Read the model definition and answer for the solid it produces. Units are mm, in the model's axes. A direction names the side the tool comes from. Give positions to 0.01 mm unless a question says otherwise; leave off trailing zeros. Loops run counter-clockwise (first coordinate to the right, second up) from the corner with the lowest first, then second, coordinate; pieces in that order, holes last. Notation, with made-up numbers: (69, 6) -> (126, 6) arc R16 cw to (126, 13) -> close; hole circle Ø8 at (89.5, -3.75). An arc over 180 degrees is marked (long way). Return JSON: item names as keys, results as strings. Group by question number.
from build123d import *

# Parameters (mm, degrees)
F0_R     = 4.25
F1_DEPTH = 3
F2_R     = 5
F3_R     = 6
F4_R     = 1
F5_SIZE  = 1


with BuildPart() as f1:
    # F0 (on Top) → F1 (new body)
    with BuildSketch(Plane.XY):
        with BuildLine():
            Line((-62.1857971695, 22.9072221785), (-52.3882933556, 32.7997051499))
            ThreePointArc((-52.3882933556, 32.7997051499), (-50.9844964361, 40.1186300293), (-48.1611355423, 47.0154365688))
            Line((-48.1611355423, 47.0154365688), (-69.9716899396, 24.9934458586))
            Line((-69.9716899396, 24.9934458586), (-62.1857971695, 22.9072221785))
        make_face()
        with BuildLine():
            ThreePointArc((-48.1611355423, 47.0154365688), (-50.9844964361, 40.1186300293), (-52.3882933556, 32.7997051499))
            Line((-52.3882933556, 32.7997051499), (-34.5789852905, 50.7816605657))
            ThreePointArc((-34.5789852905, 50.7816605657), (-28.0931597891, 55.634884838), (-20.47471121, 58.3878758514))
            ThreePointArc((-20.47471121, 58.3878758514), (-20.102300057, 64.1509445203), (-15.0399766137, 66.9302487327))
            ThreePointArc((-15.0399766137, 66.9302487327), (-34.3636079514, 61.5681900471), (-48.1611355423, 47.0154365688))
        make_face()
        with BuildLine():
            ThreePointArc((-15.0399766137, 66.9302487327), (-20.102300057, 64.1509445203), (-20.47471121, 58.3878758514))
            ThreePointArc((-20.47471121, 58.3878758514), (-17.7708422565, 58.794319571), (-15.0399766285, 58.9302487327))
            ThreePointArc((-15.0399766285, 58.9302487327), (-12.3091109856, 58.7943195724), (-9.6052420174, 58.3878758514))
            ThreePointArc((-9.6052420174, 58.3878758514), (-9.1829975469, 59.628021329), (-9.0399766137, 60.9302487327))
            ThreePointArc((-9.0399766137, 60.9302487327), (-10.7973359266, 65.1728894198), (-15.0399766137, 66.9302487327))
        make_face()
        with BuildLine():
            ThreePointArc((-13.0399766137, 60.9302487327), (-13.6257630566, 59.5160351651), (-15.0399766285, 58.9302487327))
            ThreePointArc((-15.0399766285, 58.9302487327), (-16.4541901709, 62.3444623003), (-13.0399766137, 60.9302487327))
        make_face(mode=Mode.SUBTRACT)
        with BuildLine():
            ThreePointArc((-15.0399766285, 58.9302487327), (-17.7708422565, 58.794319571), (-20.47471121, 58.3878758514))
            ThreePointArc((-20.47471121, 58.3878758514), (-15.0399766137, 54.9302487327), (-9.6052420174, 58.3878758514))
            ThreePointArc((-9.6052420174, 58.3878758514), (-12.3091109856, 58.7943195724), (-15.0399766285, 58.9302487327))
        make_face()
        with BuildLine():
            ThreePointArc((1.4030809655, 2.8767422936), (1.5045728658, 0.9401614715), (3.2006690581, 0))
            Line((3.2006690581, 0), (8.2003000527, 0))
            ThreePointArc((8.2003000527, 0), (17.7947523333, 11.3158739167), (22.25, 25.4669616943))
            ThreePointArc((22.25, 25.4669616943), (22.40748073, 27.4458247627), (22.4600233863, 29.4302487327))
            ThreePointArc((22.4600233863, 29.4302487327), (11.4765276808, 55.9467530272), (-15.0399766137, 66.9302487327))
            ThreePointArc((-15.0399766137, 66.9302487327), (-10.7973359266, 65.1728894198), (-9.0399766137, 60.9302487327))
            ThreePointArc((-9.0399766137, 60.9302487327), (-9.1829975469, 59.628021329), (-9.6052420174, 58.3878758514))
            ThreePointArc((-9.6052420174, 58.3878758514), (6.2403570467, 48.8485551745), (12.4600233863, 31.4302487327))
            ThreePointArc((12.4600233863, 31.4302487327), (12.0822423248, 26.8876459708), (10.9592786697, 22.4698511575))
            ThreePointArc((10.9592786697, 22.4698511575), (9.6768596595, 19.375042196), (8.0276528973, 16.4591275743))
            Line((8.0276528973, 16.4591275743), (1.4030809655, 2.8767422936))
        make_face()
        with BuildLine():
            ThreePointArc((22.25, 25.4669616943), (17.7947523333, 11.3158739167), (8.2003000527, 0))
            Line((8.2003000527, 0), (29.5, 0))
            ThreePointArc((29.5, 0), (37.5, 8), (29.5, 16))
            Line((29.5, 16), (27.25, 16))
            ThreePointArc((27.25, 16), (23.7144660941, 17.4644660941), (22.25, 21))
            Line((22.25, 21), (22.25, 22.4049843981))
            Line((22.25, 22.4049843981), (22.25, 25.4669616943))
        make_face()
        with Locations((29.5, 8)):
            Circle(F0_R, mode=Mode.SUBTRACT)
    extrude(amount=F1_DEPTH)

    # F2
    f2_edges = [f1.edges().sort_by_distance(p)[0] for p in [
        (-20.474711, 58.387876, 1.5),
        (-9.605242, 58.387876, 1.5),
    ]]
    fillet(f2_edges, radius=F2_R)

    # F3
    f3_edges = [f1.edges().sort_by_distance(p)[0] for p in [
        (22.25, 25.466962, 1.5),
    ]]
    fillet(f3_edges, radius=F3_R)

    # F4
    f4_edges = [f1.edges().sort_by_distance(p)[0] for p in [
        (-69.97169, 24.993446, 1.5),
        (-62.185797, 22.907222, 1.5),
    ]]
    fillet(f4_edges, radius=F4_R)

    # F5
    f5_edges = [f1.edges().sort_by_distance(p)[0] for p in [
        (25.25, 8, 3),
        (25.25, 8, 0),
    ]]
    chamfer(f5_edges, length=F5_SIZE)


solid = f1.part
1. Straight lines are drawn through the part: line 1 (Y direction, x = 29.5, z = 1.25); line 2 (X direction, y = 60, z = 2.3); line 3 (X direction, y = 32, z = 2.5). For each, find the intervals that lie inside material, in ascending order. Write a range as from..to.
2. Section A-A on x = 6 is taken. Determine the outline of the cut face in (y, z), then the cut area to 3 significant figures.
3. Which of the six approach directions +Z, -Z, +X, -X, +Y, -Y give full straight-line access (tool end or side, diameter ignored) to faces 1 (the cylindrical face through (26.13, 5.41, 1.49)), 2 (the flat face through (16, 0, 1)), 3 (the cylindrical face through (-29.74, 54.67, 1.48)), 4 (the cylindrical face through (23.75, 17.43, 1.48)), 5 (the flat face through (4.76, 9.76, 1.48))?
4. Determine the mould class of faces 6 (the flat face through (22.25, 23, 1)), 7 (the flat face through (28, 16, 1)), 8 (the flat face through (12, 41, 0)) for opening direction Y: pulls with the +Y half, pulls with the -Y half, needs draft (parallel to the pull), parting line crosses it, or undercut.
5. Section B-B on y = 8 is taken. Determine the outline of the cut face in (x, z).
6. A flat-ended cylindrical pin translates along its axis: pin 1 Ø1.1 at (x, z) = (29, 1.5) entering from +Y. Find the tip coordinate at first contact, or state that the pin passes through.
7. Section C-C on y = 35 is taken. Determine the outline of the cut face in (x, z), then the cut area to 3 significant figures.
8. Section D-D on x = -31 is taken. Determine the outline of the cut face in (y, z), then the cut area to 3 significant figures.
Completed:
{
 "1": {"line 1": "y = 0..3.75, 12.25..16", "line 2": "x = -36.76..-16.81, -13.27..6.68", "line 3": "x = -63.03..-53.18, 12.45..22.37"},
 "2": {"outline": "(0, 0) -> (12.3, 0) -> (12.3, 3) -> (0, 3) -> close; (49.14, 0) -> (60.47, 0) -> (60.47, 3) -> (49.14, 3) -> close", "area": "70.9 mm²"},
 "3": {"face 1": "+Z, -Z", "face 2": "+Z, -Z, +X, -X, -Y", "face 3": "+Z, -Z, -Y", "face 4": "+Z, -Z, +X", "face 5": "+Z, -Z, -X"},
 "4": {"face 6": "undercut", "face 7": "pulls with the +Y half", "face 8": "needs draft"},
 "5": {"outline": "(3.9, 0) -> (24.25, 0) -> (25.25, 1) -> (25.25, 2) -> (24.25, 3) -> (3.9, 3) -> close; (33.75, 1) -> (34.75, 0) -> (37.5, 0) -> (37.5, 3) -> (34.75, 3) -> (33.75, 2) -> close"},
 "6": {"pin 1": "stops at y = 16"},
 "7": {"outline": "(-60.06, 0) -> (-50.21, 0) -> (-50.21, 3) -> (-60.06, 3) -> close; (12.23, 0) -> (22.04, 0) -> (22.04, 3) -> (12.23, 3) -> close", "area": "59.0 mm²"},
 "8": {"outline": "(53.83, 0) -> (63.36, 0) -> (63.36, 3) -> (53.83, 3) -> close", "area": "28.6 mm²"}
}
